Source: CAD feature listing. Evaluate the final solid. Frame: model axes, mm. A direction names the side the tool comes from. Give positions to 0.01 mm unless a question says otherwise; leave off trailing zeros. Use CSV: the item, a comma, the result in double quotes. Start each with the question number.
1. Pin query (flat end, axial travel): P1, Ø6, axis at x = 5, y = 11.5, coming from the +Z side; P2, Ø3, axis at x = 8, z = -13, coming from the +Y side; P3, Ø8, axis at x = -8.5, z = -37, coming from the -Y side. Return the tip coordinate at first contact, or that it passes through.
2. Mould query, pull axis X, two halves, no side actions, for faces 1 (the cylindrical face through (-24.25, -3.43, 35.88)), 2 (the flat face through (10, 11, 1)), 3 (the cylindrical face through (24.29, -3.33, -60.28)). Classes: released by +X, released by -X, zero draft, split by the parting line, or undercut.
3. Reachability of faces 4 (the flat face through (-0.32, 10.98, -49.74)), 5 (the flat face through (-10, 11, 1)) from +Z, -Z, +X, -X, +Y, -Y: full face, straight path, thin tool, end or side. Return the list, or none.
4. Line query: line 1 along X through (y, z) = (4, -10.5); line 2 along Z through (x, y) = (20, -1); line 3 along Y through (x, z) = (-8.5, 15). Output: solid intervals per line, ascending. Write a range as [from, to].
from build123d import *

# Parameters (mm, degrees)
BOSS_EXTRUDE4_DEPTH      = 25
BOSS_EXTRUDE4_DEPTH_BACK = 25
SKETCH4_W                = 20
SKETCH4_H                = 75.64878903
CUT_EXTRUDE1_DEPTH       = 71.37795066
FILLET1_R                = 2.5


with BuildPart() as part:
    # Sketch5 → Boss-Extrude4 (new, two sides: drawn at the far end of the back side and taken through both)
    with BuildSketch(Plane(origin=(0, 0, 0), x_dir=(0, 0, -1), z_dir=(1, 0, 0)).offset(-BOSS_EXTRUDE4_DEPTH_BACK)):
        with BuildLine():
            Line((-37.824394515, 0), (-37.824394515, -2.5))
            Line((-37.824394515, -2.5), (-35.324394515, -5))
            add(Edge.make_bspline(
                [(-35.324394515, -5), (-13.532580845, -13.372844958), (11.79523655, -17.250489512), (59.675605485, -5)],
                knots=[0, 0, 0, 0, 1, 1, 1, 1], degree=3))
            Line((59.675605485, -5), (62.175605485, -2.5))
            Line((62.175605485, -2.5), (62.175605485, 0))
            Line((62.175605485, 0), (37.824394515, 21.5))
            Line((37.824394515, 21.5), (-37.824394515, 21.5))
            Line((-37.824394515, 21.5), (-37.824394515, 0))
        make_face()
    extrude(amount=BOSS_EXTRUDE4_DEPTH + BOSS_EXTRUDE4_DEPTH_BACK)

    # Sketch4 → Cut-Extrude1 (cut, through all)
    with BuildSketch(Plane(origin=(0, 0, 0), x_dir=(1, 0, 0), z_dir=(0, 1, 0))):
        Rectangle(SKETCH4_W, SKETCH4_H)
    extrude(amount=CUT_EXTRUDE1_DEPTH, mode=Mode.SUBTRACT)

    # Fillet1
    fillet1_edges = [part.edges().sort_by_distance(p)[0] for p in [
        (-25, -3.75, 36.574394515),
        (0, 0, -62.175605485),
        (0, -2.5, -62.175605485),
        (12.5, -5, -59.675605485),
        (12.5, -5, 35.324394515),
        (0, -2.5, 37.824394515),
        (-25, -12.695636992, -12.039484877),
        (-25, -3.75, -60.925605485),
        (25, 9.5, 37.824394515),
        (25, -3.75, 36.574394515),
        (25, -12.695636992, -12.039484877),
        (-25, -1.25, -62.175605485),
        (25, -3.75, -60.925605485),
        (25, -1.25, -62.175605485),
        (25, 10.75, -50),
        (25, 21.5, 0),
        (-25, 10.75, -50),
        (-25, 21.5, 0),
        (-25, 9.5, 37.824394515),
    ]]
    fillet(fillet1_edges, radius=FILLET1_R)


solid = part.part
Result set:
1,P1,"z = -37.82"
1,P2,"y = 0"
1,P3,"y = -10.59"
2,face 1,"released by -X"
2,face 2,"undercut"
2,face 3,"released by +X"
3,face 4,"-Z, +X, -X, +Y"
3,face 5,"+Z, +Y"
4,line 1,"[-25, -10], [10, 25]"
4,line 2,"[-62.17, 37.82]"
4,line 3,"[-10.87, 0]"
